Here's how the part is built. I have some questions about the finished solid (model axes, mm). Face numbers are marked on the shaded views. Round coordinates to 2 decimals unless told otherwise and drop trailing zeros. Write each loop counter-clockwise with the first axis right and the second up, starting at its lowest first coordinate (ties: lowest second). Pieces come first, ordered by that corner, then holes. Notation, with made-up numbers: M -38.75,84.25 L -12.75,84.25 A17 ccw -12.75,112.25 Z; hole C 9,4 d8. An arc over 180 degrees is marked long. Use one line per item in the form item = value. Start each with the question number.
Q1. We'd pull the mould along Y, two halves only. Please class the marked faces 1, 2, 3 and 4: +Y half, -Y half, draft (parallel to the pull), parting line (faces both ways), or undercut.
Q2. I want a section at B-B on y = 7.5. List the corners of the cut face in (x, z) for me.
Q3. I'm going to push flat-ended pins straight in: pin 1 Ø8 at (y, z) = (-9, 87) entering from -X; pin 2 Ø5 at (x, z) = (-17, 69) entering from +Y; pin 3 Ø3.5 at (y, z) = (12, 120.5) entering from -X; pin 4 Ø9.5 at (x, y) = (4, 2.5) entering from -Z. Where does each tip first touch, or does it pass through?
Q4. I want a section at A-A on z = 123.5. List the corners of the cut face in (x, y) for me (1 decimal).
Q5. I need wall thicknesses on line 1 along Z through (x, y) = (0, 17.9); line 2 along Y through (x, z) = (0, 118); line 3 along Y through (x, z) = (0, 37) (1 decimal). Which ranges of each line are inside material? Lowest first, please. Write a range as from..to.
Q6. I want a section at C-C on x = 18.5. List the corners of the cut face in (y, z) for me, and give its area (3 significant figures).
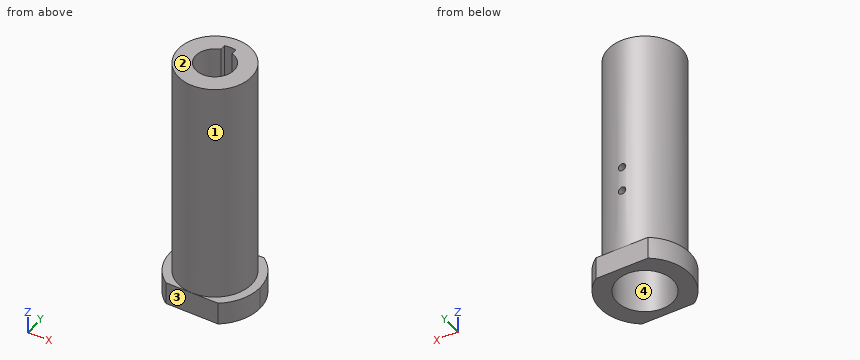
```python
from build123d import *

# Parameters (mm, degrees)
SKETCH1_R           = 20.6375
SKETCH1_R_2         = 15.875
BOSS_EXTRUDE1_DEPTH = 76.2
SKETCH2_R           = 20.6375
SKETCH2_R_2         = 13.9954
BOSS_EXTRUDE2_DEPTH = 63.5
BOSS_EXTRUDE3_DEPTH = 12.7
BOSS_EXTRUDE4_START = -63.5
BOSS_EXTRUDE4_DEPTH = 63.5
SKETCH5_R           = 2.0828
CUT_EXTRUDE1_DEPTH  = 13.208


with BuildPart() as part:
    # Sketch1 → Boss-Extrude1 (new body)
    with BuildSketch(Plane.XY):
        with Locations(Location((0, 0, 0), (0, 0, 180))):
            Circle(SKETCH1_R)
        with Locations(Location((0, 0, 0), (0, 0, 180))):
            Circle(SKETCH1_R_2, mode=Mode.SUBTRACT)
    extrude(amount=BOSS_EXTRUDE1_DEPTH)

    # Sketch2 → Boss-Extrude2 (add)
    with BuildSketch(Plane.XY.offset(76.2)):
        with Locations(Location((0, 0, 0), (0, 0, 180))):
            Circle(SKETCH2_R)
        Circle(SKETCH2_R_2, mode=Mode.SUBTRACT)
    extrude(amount=BOSS_EXTRUDE2_DEPTH)

    # Sketch3 → Boss-Extrude3 (add)
    with BuildSketch(Plane.XY):
        with BuildLine():
            ThreePointArc((25.4, 0), (22.597159577, 11.598636949), (14.807214247, 20.6375))
            Line((14.807214247, 20.6375), (0, 20.6375))
            ThreePointArc((0, 20.6375), (14.592916197, 14.592916197), (20.6375, 0))
            ThreePointArc((20.6375, 0), (14.592916219, -14.592916175), (6.2e-08, -20.6375))
            Line((6.2e-08, -20.6375), (14.807214247, -20.6375))
            ThreePointArc((14.807214247, -20.6375), (22.597159577, -11.598636949), (25.4, 0))
        make_face()
        with BuildLine():
            ThreePointArc((6.2e-08, -20.6375), (-20.6375, -3.1e-08), (0, 20.6375))
            Line((0, 20.6375), (-14.807214247, 20.6375))
            ThreePointArc((-14.807214247, 20.6375), (-25.4, 0), (-14.807214247, -20.6375))
            Line((-14.807214247, -20.6375), (6.2e-08, -20.6375))
        make_face()
    extrude(amount=BOSS_EXTRUDE3_DEPTH)

    # Sketch4 → Boss-Extrude4 (add)
    with BuildSketch(Plane.XY.offset(139.7).offset(BOSS_EXTRUDE4_START)):
        with BuildLine():
            ThreePointArc((10.8077, 0), (-6.422302227, -8.692549304), (-3.175, 10.330815761))
            Line((-3.175, 10.330815761), (-3.175, 13.630502418))
            ThreePointArc((-3.175, 13.630502418), (-8.701604052, -10.961446441), (13.9954, 0))
            ThreePointArc((13.9954, 0), (10.961446441, 8.701604052), (3.175, 13.630502418))
            Line((3.175, 13.630502418), (3.175, 10.330815761))
            ThreePointArc((3.175, 10.330815761), (8.692549304, 6.422302227), (10.8077, 0))
        make_face()
    extrude(amount=BOSS_EXTRUDE4_DEPTH)

    # Sketch5 → Cut-Extrude1 (cut)
    with BuildSketch(Plane(origin=(0, 20.6375, 0), x_dir=(1, 0, 0), z_dir=(0, 1, 0))):
        with Locations(Location((0, -61.9125, 0), (0, 0, 270))):
            Circle(SKETCH5_R)
        with Locations(Location((0, -47.625, 0), (0, 0, 270))):
            Circle(SKETCH5_R)
    extrude(amount=-CUT_EXTRUDE1_DEPTH, mode=Mode.SUBTRACT)


solid = part.part
```
Reported:
q1.face_1 = parting line
q1.face_2 = draft
q1.face_3 = -Y half
q1.face_4 = undercut
q2.outline = M -24.27,0 L -13.99,0 L -13.99,76.2 L -7.78,76.2 L -7.78,139.7 L -19.23,139.7 L -19.23,12.7 L -24.27,12.7 Z; M 7.78,76.2 L 13.99,76.2 L 13.99,0 L 24.27,0 L 24.27,12.7 L 19.23,12.7 L 19.23,139.7 L 7.78,139.7 Z
q3.pin_1 = -20.02
q3.pin_2 = 14.69
q3.pin_3 = -17.91
q3.pin_4 = through
q4.outline = C 0,0 d41.3; hole M -3.2,10.3 A10.8 ccw long 3.2,10.3 L 3.2,13.6 A14 ccw -3.2,13.6 Z
q5.line_1 = 0..45.54, 49.71..59.83, 64..139.7
q5.line_2 = -20.64..-10.81, 14..20.64
q5.line_3 = -20.6..-15.9, 15.9..20.6
q6.outline = M -17.4,0 L 17.4,0 L 17.4,12.7 L 9.15,12.7 L 9.15,139.7 L -9.15,139.7 L -9.15,12.7 L -17.4,12.7 Z
q6.area = 2,770 mm^2
